```python
from build123d import *

# Parameters (mm, degrees)
SKETCH_1_R          = 10
EXTRUDE_1_DEPTH     = 2
SKETCH_2_R          = 4
EXTRUDE_2_DEPTH     = 2
SKETCH_3_R          = 3.05
CUT_EXTRUDE_1_DEPTH = 3.5
SKETCH_4_R          = 0.75
CUT_EXTRUDE_2_DEPTH = 15.282856857


with BuildPart() as part:
    # 草图1 → 凸台-拉伸1 (new body)
    with BuildSketch(Plane.XY):
        Circle(SKETCH_1_R)
    extrude(amount=EXTRUDE_1_DEPTH)

    # 草图2 → 凸台-拉伸2 (add)
    with BuildSketch(Plane(origin=(0, 0, 0), x_dir=(-1, 0, 0), z_dir=(0, 0, -1))):
        Circle(SKETCH_2_R)
    extrude(amount=EXTRUDE_2_DEPTH)

    # 草图3 → 切除-拉伸1 (cut)
    with BuildSketch(Plane(origin=(0, 0, -2), x_dir=(-1, 0, 0), z_dir=(0, 0, -1))):
        Circle(SKETCH_3_R)
    extrude(amount=-CUT_EXTRUDE_1_DEPTH, mode=Mode.SUBTRACT)

    # 草图4 → 切除-拉伸2 (cut, through all)
    with BuildSketch(Plane(origin=(0, 0, 0), x_dir=(-1, 0, 0), z_dir=(0, 0, -1))):
        with Locations((0, 7)):
            Circle(SKETCH_4_R)
        with Locations((7, 0)):
            Circle(SKETCH_4_R)
        with Locations((0, -7)):
            Circle(SKETCH_4_R)
        with Locations((-7, 0)):
            Circle(SKETCH_4_R)
    extrude(amount=-CUT_EXTRUDE_2_DEPTH, mode=Mode.SUBTRACT)


solid = part.part
```
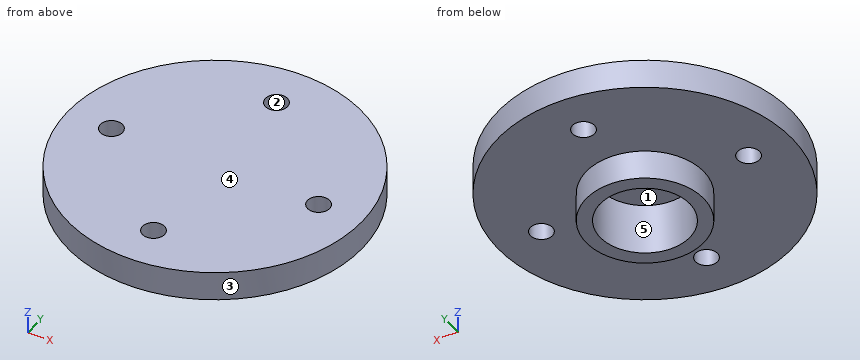
The listing builds one solid part. Answer for the finished solid, in the listing's coordinates (mm). Face numbers are marked on the shaded views. A direction names the side the tool comes from. Coordinates: 2 decimals unless noted, no trailing zeros. Loops run counter-clockwise (first coordinate to the right, second up) from the corner with the lowest first, then second, coordinate; pieces in that order, holes last. Notation, with made-up numbers: (44.5, -19.75) - (69.5, -19.75) arc R30 ccw to (69.5, 7.25) - close; hole circle Ø6 at (31.5, 21). An arc over 180 degrees is marked (long way). Use a Markdown table: item, result. Add a question column.
1) For the marked faces 1 and 2, determine the directions among +Z, -Z, +X, -X, +Y, -Y from which every point of the face is accessible in a straight line to the end or side of a thin tool.
2) Given pin 1 (1.7 mm diameter, centred on x = 7, y = 0, fed in from -Z); pin 2 (3 mm diameter, centred on x = 0, y = -0.5, fed in from -Z), each flat-ended and moving along its own axis, determine where each tip first touches the part or whether it passes through.
3) The part is cut by section C-C, the plane z = -1.2. Give the vertices of the cut face in (x, y), and give its area (3 significant figures).
4) The part is cut by section D-D, the plane x = 6.5. Give the vertices of the cut face in (y, z), and give its area (3 significant figures).
5) The mould has two halves that part along Y. Classify the marked faces 3, 4 and 5: released by +Y, released by -Y, zero draft, split by the parting line, or undercut.
6) The part is cut by section A-A, the plane y = 0. Give the vertices of the cut face in (x, z), and give its area (4 significant figures).
7) Find the intervals of material crossed by line 1 (Y direction, x = 0, z = 0.15); line 2 (Z direction, x = 2, y = -8); line 3 (Y direction, x = -7.5, z = 0.25), in increasing order.
Here are the results:
| question | item | result |
|---|---|---|
| 1 | face 1 | -Z |
| 1 | face 2 | +Z, -Z |
| 2 | pin 1 | stops at z = 0 |
| 2 | pin 2 | stops at z = 1.5 |
| 3 | outline | circle Ø8 at (0, 0); hole circle Ø6.1 at (0, 0) |
| 3 | area | 21.0 mm^2 |
| 4 | outline | (-7.6, 0) - (-0.56, 0) - (-0.56, 2) - (-7.6, 2) - close; (0.56, 0) - (7.6, 0) - (7.6, 2) - (0.56, 2) - close |
| 4 | area | 28.2 mm^2 |
| 5 | face 3 | split by the parting line |
| 5 | face 4 | zero draft |
| 5 | face 5 | undercut |
| 6 | outline | (-10, 0) - (-7.75, 0) - (-7.75, 2) - (-10, 2) - close; (-6.25, 0) - (-4, 0) - (-4, -2) - (-3.05, -2) - (-3.05, 1.5) - (3.05, 1.5) - (3.05, -2) - (4, -2) - (4, 0) - (6.25, 0) - (6.25, 2) - (-6.25, 2) - close; (7.75, 0) - (10, 0) - (10, 2) - (7.75, 2) - close |
| 6 | area | 28.65 mm^2 |
| 7 | line 1 | y = -10 to -7.75, -6.25 to -3.05, 3.05 to 6.25, 7.75 to 10 |
| 7 | line 2 | z = 0 to 2 |
| 7 | line 3 | y = -6.61 to -0.56, 0.56 to 6.61 |
